Can you work these out from the model? Positions are in its coordinate system, mm. Coordinates: 2 decimals unless noted, no trailing zeros. Order: outer loops, then holes, each group sorted by start corner. A loop starts at its lowest first (then second) coordinate and runs counter-clockwise, first axis right, second up. Notation, with made-up numbers: (11, 62) - (70, 62) arc R36 ccw to (70, 100) - close; hole circle Ø4 at (41, 24). An arc over 180 degrees is marked (long way). Use a Markdown table: item, result. Add a question column.
(1) I want a section at C-C (x = 11). List the corners of the cut face in (y, z) for me (1 decimal).
(2) I want a section at A-A (z = -31). List the corners of the cut face in (x, y) for me (1 decimal), and give its area (3 significant figures).
(3) For pin 1 Ø12 at (y, z) = (0.5, 35) entering from +X; pin 2 Ø14 at (x, z) = (9, 13) entering from +Y; pin 3 Ø7 at (y, z) = (-5.5, 72) entering from -X; pin 4 Ø4 at (x, z) = (-14.29, -142.94) entering from -Y (3 decimals), each with a flat end and sliding along its axis, tell me the tip position at first contact or that it passes through.
(4) I want a section at B-B (y = -4). List the corners of the cut face in (x, z) for me.
(5) If I drill on L1, parallel to X at y = -10, z = -20.5; L2, parallel to Y at x = 11.5, z = -15.5 (1 decimal); L3, parallel to X at y = 0, z = -50, over which ranges is the centre line in solid material (lowest first)? Write a range as [from, to].
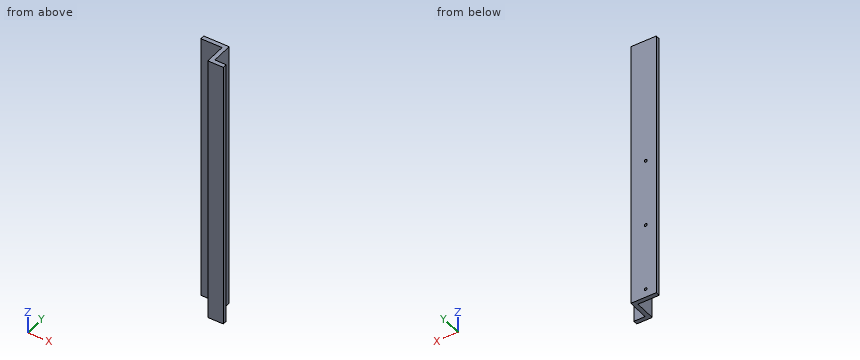
```python
from build123d import *

# Parameters (mm, degrees)
BOSS_EXTRUDE1_DEPTH      = 152.4
BOSS_EXTRUDE1_DEPTH_BACK = 152.4
SKETCH6_R                = 1.5875
CUT_EXTRUDE1_DEPTH       = 4.7625


with BuildPart() as part:
    # Sketch3 → Boss-Extrude1 (new, two sides: drawn at the far end of the back side and taken through both)
    with BuildSketch(Plane.XY.offset(-BOSS_EXTRUDE1_DEPTH_BACK)):
        Polygon((15.08125, -9.525), (15.08125, -14.2875), (-2.38125, -14.2875), (-2.38125, 9.525), (-26.19375, 9.525), (-26.19375, 14.2875), (2.38125, 14.2875), (2.38125, -9.525), align=None)
    extrude(amount=BOSS_EXTRUDE1_DEPTH + BOSS_EXTRUDE1_DEPTH_BACK)

    # Sketch6 → Cut-Extrude1 (cut)
    with BuildSketch(Plane.XZ.offset(-9.525)):
        with Locations(Location((-14.2875, 9.463870403, 0), (0, 0, 270))):
            Circle(SKETCH6_R)
        with Locations(Location((-14.2875, -66.736129597, 0), (0, 0, 270))):
            Circle(SKETCH6_R)
        with Locations(Location((-14.2875, -142.936129597, 0), (0, 0, 270))):
            Circle(SKETCH6_R)
    extrude(amount=-CUT_EXTRUDE1_DEPTH, mode=Mode.SUBTRACT)


solid = part.part
```
Answers follow:
| question | item | result |
|---|---|---|
| 1 | outline | (-14.3, -152.4) - (-9.5, -152.4) - (-9.5, 152.4) - (-14.3, 152.4) - close |
| 2 | outline | (-26.2, 9.5) - (-2.4, 9.5) - (-2.4, -14.3) - (15.1, -14.3) - (15.1, -9.5) - (2.4, -9.5) - (2.4, 14.3) - (-26.2, 14.3) - close |
| 2 | area | 310 mm² |
| 3 | pin 1 | stops at x = 2.38 |
| 3 | pin 2 | stops at y = 14.29 |
| 3 | pin 3 | stops at x = -2.38 |
| 3 | pin 4 | stops at y = 9.525 |
| 4 | outline | (-2.38, -152.4) - (2.38, -152.4) - (2.38, 152.4) - (-2.38, 152.4) - close |
| 5 | L1 | x = [-2.38, 15.08] |
| 5 | L2 | y = [-14.3, -9.5] |
| 5 | L3 | x = [-2.38, 2.38] |
